Geometry: final body of the model. Coordinates: model frame, mm. Give positions to 0.01 mm unless a question says otherwise; leave off trailing zeros. Loops run counter-clockwise (first coordinate to the right, second up) from the corner with the lowest first, then second, coordinate; pieces in that order, holes last. Notation, with made-up numbers: (-20, -38) -> (10, -38) arc R22 ccw to (10, -6) -> close; hole circle Ø11 at (-39, 52). An arc over 180 degrees is marked (long way). Answer in a Markdown table with one row per item. Add a question column.
1) Line query: line 1 (X direction, y = -3.95, z = 20.9); line 2 (Z direction, x = -12.5, y = -5.1); line 3 (Z direction, x = 15, y = -4.15). Output: solid intervals per line, ascending. Write a range as from..to.
2) First-contact query: P1, Ø1.5, axis at x = 10, y = -5, coming from the +Z side; P2, Ø0.9, axis at y = -5, z = -6, coming from the +X side; P3, Ø1.5, axis at x = 13.5, y = -4, coming from the -Z side. Flat tips, straight axial feed; report the tip coordinate or a pass-through.
3) Section query C-C (z = 0). Return the cut outline in (x, y), plus the area to 3 significant figures.
4) Section query A-A (z = 20.9). Return the cut outline in (x, y), plus the area to 3 significant figures.
5) Section query D-D (y = -3.45). Return the cut outline in (x, z), plus the area to 3 significant figures.
6) Section query B-B (x = -12.5). Return the cut outline in (y, z).
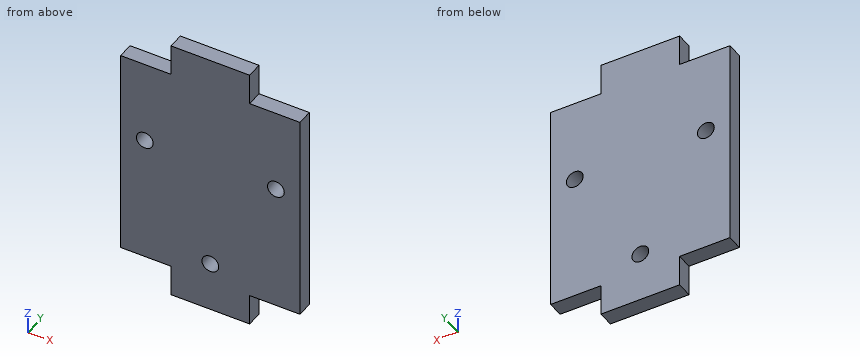
```python
from build123d import *

# Parameters (mm, degrees)
ESBO_O1_R                = 1.6
RESSALTO_EXTRUS_O1_DEPTH = 3


with BuildPart() as part:
    # Esboço1 → Ressalto-extrusão1 (new body)
    with BuildSketch(Plane.XZ.offset(6)):
        Polygon((17.1, 36.9), (7.5, 36.9), (7.5, 42.9), (-7.5, 42.9), (-7.5, 36.9), (-17.1, 36.9), (-17.1, -3.6), (-7.5, -3.6), (-7.5, -9.6), (7.5, -9.6), (7.5, -3.6), (17.1, -3.6), align=None)
        with Locations(Location((-12.5, 20.9, 0), (0, 0, 90))):
            Circle(ESBO_O1_R, mode=Mode.SUBTRACT)
        with Locations(Location((0, 0, 0), (0, 0, 90))):
            Circle(ESBO_O1_R, mode=Mode.SUBTRACT)
        with Locations(Location((12.5, 20.9, 0), (0, 0, 90))):
            Circle(ESBO_O1_R, mode=Mode.SUBTRACT)
    extrude(amount=-RESSALTO_EXTRUS_O1_DEPTH)


solid = part.part
```
Evaluation:
| question | item | result |
|---|---|---|
| 1 | line 1 | -17.1..-14.1, -10.9..10.9, 14.1..17.1 |
| 1 | line 2 | -3.6..19.3, 22.5..36.9 |
| 1 | line 3 | -3.6..36.9 |
| 2 | P1 | z = 36.9 |
| 2 | P2 | x = 7.5 |
| 2 | P3 | z = -3.6 |
| 3 | outline | (-17.1, -6) -> (-1.6, -6) -> (-1.6, -3) -> (-17.1, -3) -> close; (1.6, -6) -> (17.1, -6) -> (17.1, -3) -> (1.6, -3) -> close |
| 3 | area | 93.0 mm² |
| 4 | outline | (-17.1, -6) -> (-14.1, -6) -> (-14.1, -3) -> (-17.1, -3) -> close; (-10.9, -6) -> (10.9, -6) -> (10.9, -3) -> (-10.9, -3) -> close; (14.1, -6) -> (17.1, -6) -> (17.1, -3) -> (14.1, -3) -> close |
| 4 | area | 83.4 mm² |
| 5 | outline | (-17.1, -3.6) -> (-7.5, -3.6) -> (-7.5, -9.6) -> (7.5, -9.6) -> (7.5, -3.6) -> (17.1, -3.6) -> (17.1, 36.9) -> (7.5, 36.9) -> (7.5, 42.9) -> (-7.5, 42.9) -> (-7.5, 36.9) -> (-17.1, 36.9) -> close; hole circle Ø3.2 at (-12.5, 20.9); hole circle Ø3.2 at (0, 0); hole circle Ø3.2 at (12.5, 20.9) |
| 5 | area | 1,540 mm² |
| 6 | outline | (-6, -3.6) -> (-3, -3.6) -> (-3, 19.3) -> (-6, 19.3) -> close; (-6, 22.5) -> (-3, 22.5) -> (-3, 36.9) -> (-6, 36.9) -> close |
